Design review of the part built by this model. Coordinates are the model's own, in mm. A direction names the side the tool comes from. Coordinates: 2 decimals unless noted, no trailing zeros. Loops run counter-clockwise (first coordinate to the right, second up) from the corner with the lowest first, then second, coordinate; pieces in that order, holes last. Notation, with made-up numbers: M 36.25,-22.5 L 84.25,-22.5 A16 cw 84.25,-0.5 Z; hole C 12.5,23 d8. An arc over 180 degrees is marked long. Answer as a JSON object with one key per item and string values. Group by question number.
1. Draft analysis for pull direction Z (two halves, no side actions). For faces 5 (the flat face through (38, 69, 142.113)), 6 (the flat face through (84.897, 80, -129)), 7 (the flat face through (-165, 0, -16)), state which applies: +Z half, -Z half, draft (parallel to the pull), parting line (faces both ways), or undercut.
2. Consider section B-B (x = -31.5). State the section outline as (y, z) points (3 decimals).
3. Consider section A-A (y = 46.5). State the section outline as (x, z) points.
4. Consider section D-D (z = 33.5). State the section outline as (x, y) points.
5. Insertion check: pin 1 (12 mm diameter, centred on x = 51, y = 130, fed in from +Z); pin 2 (3 mm diameter, centred on x = 13, z = 138.5, fed in from -Y); pin 3 (5 mm diameter, centred on x = 24.5, z = -123.5, fed in from -Y); pin 4 (8 mm diameter, centred on x = -94, y = 47, fed in from -Z). Each pin has a flat end and moves straight along its axis. Give the tip position at first contact, or say it passes through.
6. To check wall thickness, follow probe 1 along X at (y, z) = (76.5, -133); probe 2 along X at (y, z) = (37.5, 16.5); probe 3 along X at (y, z) = (88, -20.5). State the ranges of each line that lie inside material, in increasing order.
7. Machinability: for faces 1 (the flat face through (-30, 82, -134.267)), 2 (the flat face through (38, 104, 135.763)), 3 (the flat face through (-161.163, 39, -16)), 4 (the cylindrical face through (41.15, 85.28, -125.39)), which of the approach directions +Z, -Z, +X, -X, +Y, -Y give a long, thin tool a straight path to every point of the face, cutting with its end or side? Answer none if there is none.
from build123d import *

# Parameters (mm, degrees)
SKETCH1_W               = 416.08
SKETCH1_H               = 314.48
BOSS_EXTRUDE2_DEPTH     = 152.4
SKETCH2_W               = 403.38
SKETCH2_H               = 308.13
CUT_EXTRUDE1_DEPTH      = 339.705913999
CUT_EXTRUDE2_DEPTH      = 476.456316699
CUT_EXTRUDE3_REACH      = 430.846
SKETCH4_W               = 111.28
SKETCH4_H               = 63.5
SKETCH5_W               = 403.38
SKETCH5_H               = 12.7
BOSS_EXTRUDE3_DEPTH     = 308.13
SKETCH6_W               = 377.98
SKETCH6_H               = 231.93
CUT_EXTRUDE4_DEPTH      = 6.35
CUT_EXTRUDE5_DEPTH      = 314.544954796
CUT_EXTRUDE5_DEPTH_BACK = 314.544954796
FILLET2_R               = 12.7
BOSS_EXTRUDE4_REACH     = 382.621
SKETCH8_R               = 1.905


with BuildPart() as part:
    # Sketch1 → Boss-Extrude2 (new body)
    with BuildSketch(Plane(origin=(0, 0, 0), x_dir=(1, 0, 0), z_dir=(0, 1, 0))):
        with Locations((40.527, 15.127)):
            Rectangle(SKETCH1_W, SKETCH1_H)
    extrude(amount=BOSS_EXTRUDE2_DEPTH)

    # Sketch2 → Cut-Extrude1 (cut, through all)
    with BuildSketch(Plane(origin=(0, 152.4, 0), x_dir=(1, 0, 0), z_dir=(0, 1, 0))):
        with Locations((40.527, 18.302)):
            Rectangle(SKETCH2_W, SKETCH2_H)
    extrude(amount=-CUT_EXTRUDE1_DEPTH, mode=Mode.SUBTRACT)

    # Sketch3 → Cut-Extrude2 (cut, through all)
    with BuildSketch(Plane(origin=(248.567, 0, 0), x_dir=(0, 0, -1), z_dir=(1, 0, 0))):
        with BuildLine():
            Line((-142.113, 114.3), (-142.113, 152.4))
            Line((-142.113, 152.4), (172.367, 152.4))
            Line((172.367, 152.4), (-65.913, 139.7))
            ThreePointArc((-65.913, 139.7), (-105.728307199, 132.145921598), (-142.113, 114.3))
        make_face()
    extrude(amount=-CUT_EXTRUDE2_DEPTH, mode=Mode.SUBTRACT)

    # Sketch4 → Cut-Extrude3 (cut, up to next)
    with BuildSketch(Plane.XY.offset(142.113), mode=Mode.PRIVATE) as cut_extrude3_sk1:
        with Locations((40.527, 31.75)):
            Rectangle(SKETCH4_W, SKETCH4_H)
    cut_extrude3_tool1 = extrude(cut_extrude3_sk1.sketch, amount=-CUT_EXTRUDE3_REACH, mode=Mode.PRIVATE) & part.part
    add(cut_extrude3_tool1.solids().sort_by_distance((40.527, 31.75, 142.113))[0], mode=Mode.SUBTRACT)

    # Sketch5 → Boss-Extrude3 (add)
    with BuildSketch(Plane(origin=(0, 0, 135.763), x_dir=(-1, 0, 0), z_dir=(0, 0, -1))):
        with Locations((-40.527, 82.55)):
            Rectangle(SKETCH5_W, SKETCH5_H)
    extrude(amount=BOSS_EXTRUDE3_DEPTH)

    # Sketch6 → Cut-Extrude4 (cut)
    with BuildSketch(Plane(origin=(0, 88.9, 0), x_dir=(1, 0, 0), z_dir=(0, 1, 0))):
        with Locations((40.527, 5.602)):
            Rectangle(SKETCH6_W, SKETCH6_H)
    extrude(amount=-CUT_EXTRUDE4_DEPTH, mode=Mode.SUBTRACT)

    # Sketch7 → Cut-Extrude5 (cut, two sides: drawn at the far end of the back side and taken through both)
    with BuildSketch(Plane(origin=(0, 82.55, 0), x_dir=(1, 0, 0), z_dir=(0, 1, 0)).offset(-CUT_EXTRUDE5_DEPTH_BACK)):
        Polygon((-54.643, 134.267), (-3.843, 134.267), (-3.843, 121.567), (84.897, 121.567), (84.897, 134.267), (135.697, 134.267), (135.697, 121.567), (224.437, 121.567), (224.437, -105.283), (-143.383, -105.283), (-143.383, 121.567), (-54.643, 121.567), align=None)
    extrude(amount=CUT_EXTRUDE5_DEPTH + CUT_EXTRUDE5_DEPTH_BACK, mode=Mode.SUBTRACT)

    # Fillet2
    fillet2_edges = [part.edges().sort_by_distance(p)[0] for p in [
        (182.607, 88.9, -121.567),
        (40.527, 88.9, -121.567),
        (-101.553, 88.9, -121.567),
    ]]
    fillet(fillet2_edges, radius=FILLET2_R - 0.0001)  # a hair under: the kernel refuses the full size

    # Boss-Extrude4: up to this face of the body (flat: up to its plane)
    boss_extrude4_end = Plane(part.part.faces().sort_by_distance((135.697, 81.590060551, -128.876939449))[0])
    # Sketch8 → Boss-Extrude4 (add, up to the picked face)
    with BuildSketch(Plane(origin=(-54.643, 0, 0), x_dir=(0, 0, -1), z_dir=(1, 0, 0)), mode=Mode.PRIVATE) as boss_extrude4_sk1:
        with Locations(Location((127.917, 82.55, 0), (0, 0, 180))):
            Circle(SKETCH8_R)
    boss_extrude4_tool1 = split(extrude(boss_extrude4_sk1.sketch, amount=BOSS_EXTRUDE4_REACH, mode=Mode.PRIVATE), bisect_by=boss_extrude4_end, keep=Keep.BOTH, mode=Mode.PRIVATE)
    add(boss_extrude4_tool1.solids().sort_by(Axis((-54.643, 82.55, -127.917), (1, 0, 0)))[0])


solid = part.part
Findings below:
{
 "1": {"face 5": "+Z half", "face 6": "undercut", "face 7": "draft"},
 "2": {"outline": "M 0,135.763 L 76.2,135.763 L 76.2,105.283 L 82.55,105.283 L 82.55,110.363 L 88.9,110.363 L 88.9,135.763 L 118.329,135.763 A151.386 ccw 114.3,142.113 L 0,142.113 Z; M 76.2,-172.367 L 88.9,-172.367 L 88.9,-134.267 L 76.2,-134.267 Z; C 82.55,-127.917 d3.81"},
 "3": {"outline": "M -167.51,-172.37 L -161.16,-172.37 L -161.16,135.76 L -15.11,135.76 L -15.11,142.11 L -167.51,142.11 Z; M 96.17,135.76 L 242.22,135.76 L 242.22,-172.37 L 248.57,-172.37 L 248.57,142.11 L 96.17,142.11 Z"},
 "4": {"outline": "M -167.51,0 L -161.16,0 L -161.16,76.2 L -143.38,76.2 L -143.38,82.55 L -148.46,82.55 L -148.46,88.9 L -161.16,88.9 L -161.16,141.43 L -167.51,141.43 Z; M 224.44,76.2 L 242.22,76.2 L 242.22,0 L 248.57,0 L 248.57,141.43 L 242.22,141.43 L 242.22,88.9 L 229.52,88.9 L 229.52,82.55 L 224.44,82.55 Z"},
 "5": {"pin 1": "passes through", "pin 2": "stops at y = 63.5", "pin 3": "stops at y = 76.2", "pin 4": "stops at z = 135.76"},
 "6": {"probe 1": "x = -167.51 to -54.64, -3.84 to 84.9, 135.7 to 248.57", "probe 2": "x = -167.51 to -161.16, 242.22 to 248.57", "probe 3": "x = -167.51 to -148.46, 229.52 to 248.57"},
 "7": {"face 1": "+Y, -Y", "face 2": "-Z, +Y", "face 3": "-Z, -Y", "face 4": "+Y"}
}
